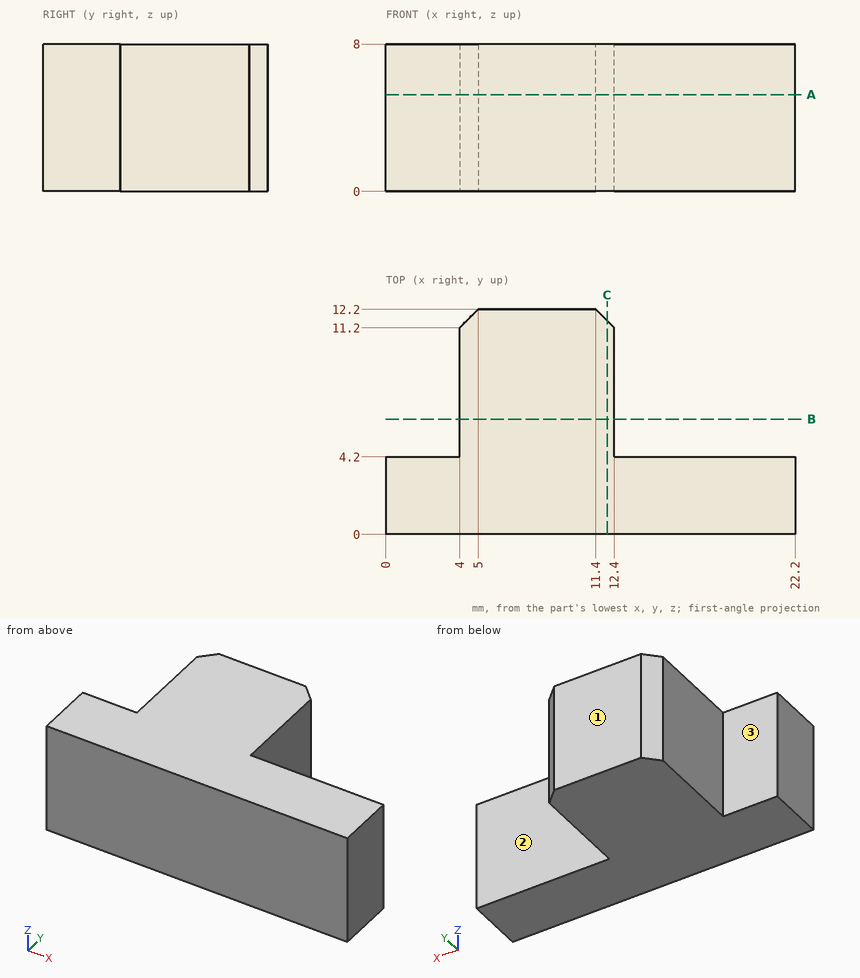
Part print with two shaded views. Sizes in mm from the minimum x, y, z corner. A direction names the side the tool comes from. Give positions to 0.01 mm unless a question says otherwise; leave off trailing zeros. Order: outer loops, then holes, each group sorted by start corner. A loop starts at its lowest first (then second) coordinate and runs counter-clockwise, first axis right, second up.
1) 3-axis set-ups, long thin cutter, end or side, ignore diameter. For the marked faces 1, 2 and 3: which of +Z, -Z, +X, -X, +Y, -Y reach the whole face in a straight line?
2) Saw through at B-B, the plane y = 6.25. Write the cut outline in (x, z).
3) Wall check: probe 1 along Y at (x, z) = (18.75, 4.5); probe 2 along X at (y, z) = (9, 2.75). Give the ranges that are in metal, low to high.
4) Pin check, flat tips, straight feed: pin 1 (1.2 mm diameter, centred on x = 1, z = 2, fed in from +Y); pin 2 (1 mm diameter, centred on y = 10.5, z = 4.5, fed in from +X); pin 3 (2 mm diameter, centred on y = 8, z = 4, fed in from -X). Stop position of each tip, or through.
5) Saw through at A-A, the plane z = 5.25. Write the cut outline in (x, y), then the cut area to 3 significant figures.
6) Saw through at C-C, the plane x = 12. Write the cut outline in (y, z), then the cut area to 3 significant figures.
Computed:
1. face 1: +Z, -Z, +X, -X, +Y
1. face 2: +Z, -Z, +X, +Y
1. face 3: +Z, -Z, -X, +Y
2. outline: (4, 0) - (12.4, 0) - (12.4, 8) - (4, 8) - close
3. probe 1: y = 0 to 4.2
3. probe 2: x = 4 to 12.4
4. pin 1: stops at y = 4.2
4. pin 2: stops at x = 12.4
4. pin 3: stops at x = 4
5. outline: (0, 0) - (22.2, 0) - (22.2, 4.2) - (12.4, 4.2) - (12.4, 11.2) - (11.4, 12.2) - (5, 12.2) - (4, 11.2) - (4, 4.2) - (0, 4.2) - close
5. area: 159 mm2
6. outline: (0, 0) - (11.6, 0) - (11.6, 8) - (0, 8) - close
6. area: 92.8 mm2
